```python
from build123d import *
from build123d import SkipClean  # not in build123d's __all__

# Parameters (mm, degrees)
F0_R     = 8.89
F0_R_2   = 5.969
F3_R     = 7.62
F3_R_2   = 5.969
F4_R     = 7.62
F4_R_2   = 5.969
F5_DEPTH = 17.78


with BuildPart() as f2:
    # F2: sweep along a path in F1
    with BuildLine(Plane.XY) as f2_path:
        Line((0, 0), (0, 12.7))
        ThreePointArc((0, 12.7), (12.7, 25.4), (25.4, 12.7))
        Line((25.4, 12.7), (25.4, 0))
    # F0 (on Front) → F2 (sweep)
    with BuildSketch(Plane.XZ):
        Circle(F0_R)
        Circle(F0_R_2, mode=Mode.SUBTRACT)
    sweep(path=f2_path.line)

    # F3 (on face) + F4 (on face) → F5 (join)
    with BuildSketch(Plane.XZ):
        Circle(F3_R)
        Circle(F3_R_2, mode=Mode.SUBTRACT)
    with BuildSketch(Plane.XZ):
        with Locations((25.4, 0)):
            Circle(F4_R)
        with Locations((25.4, 0)):
            Circle(F4_R_2, mode=Mode.SUBTRACT)
    with SkipClean():  # cleaning this boolean's faces spoils the solid; the shape is the same uncleaned
        extrude(amount=F5_DEPTH)


solid = f2.part
```
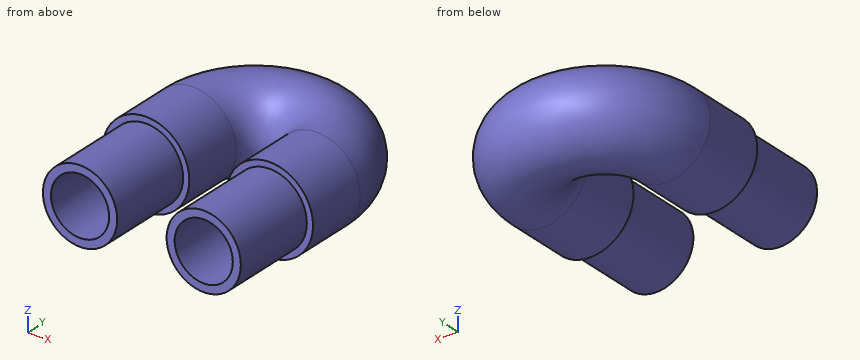
Part model, mm, in its own coordinate system. Give positions to 0.01 mm unless a question says otherwise; leave off trailing zeros. Loops run counter-clockwise (first coordinate to the right, second up) from the corner with the lowest first, then second, coordinate; pieces in that order, holes last. Notation, with made-up numbers: M -21,32.5 L 6,32.5 A16 ccw 6,52.5 Z; hole C -14,51.5 d10. An arc over 180 degrees is marked long. Return JSON: item names as keys, results as strings.
1) Flat gauge pins, fed straight in: pin 1 Ø10 at (x, z) = (5.5, -2.5) entering from +Y; pin 2 Ø1.5 at (x, z) = (28.5, -0.5) entering from -Y; pin 3 Ø6 at (y, z) = (18, -6) entering from +X; pin 4 Ø2 at (x, y) = (9, -3) entering from -Z. Where does each tip first touch, or does it go through?
Calculated:
{"pin 1": "stops at y = 34.12", "pin 2": "stops at y = 21.29", "pin 3": "stops at x = 33.27", "pin 4": "passes through"}
2) Saw through at A-A, the plane z = 0. List the corners of the cut face in (x, y).
Calculated:
{"outline": "M -8.89,0 L -7.62,0 L -7.62,-17.78 L -5.97,-17.78 L -5.97,12.7 A18.67 cw 31.37,12.7 L 31.37,-17.78 L 33.02,-17.78 L 33.02,0 L 34.29,0 L 34.29,12.7 A21.59 ccw -8.89,12.7 Z; M 5.97,-17.78 L 7.62,-17.78 L 7.62,0 L 8.89,0 L 8.89,12.7 A3.81 cw 16.51,12.7 L 16.51,0 L 17.78,0 L 17.78,-17.78 L 19.43,-17.78 L 19.43,12.7 A6.73 ccw 5.97,12.7 Z"}
3) Saw through at C-C, the plane z = 3.5. List the corners of the cut face in (x, y).
Calculated:
{"outline": "M -8.17,0 L -6.77,0 L -6.77,-17.78 L -4.84,-17.78 L -4.84,12.7 A17.54 cw 30.24,12.7 L 30.24,-17.78 L 32.17,-17.78 L 32.17,0 L 33.57,0 L 33.57,12.7 A20.87 ccw -8.17,12.7 Z; M 4.84,-17.78 L 6.77,-17.78 L 6.77,0 L 8.17,0 L 8.17,12.7 A4.53 cw 17.23,12.7 L 17.23,0 L 18.63,0 L 18.63,-17.78 L 20.56,-17.78 L 20.56,12.7 A7.86 ccw 4.84,12.7 Z"}
4) Drill centre lines: line 1 (X direction, y = 3, z = 1.25); line 2 (X direction, y = -2, z = 3.25); line 3 (X direction, y = 18.5, z = -1). Where is each one in solid material? Low to high.
Calculated:
{"line 1": "x = -8.8 to -5.84, 5.84 to 8.8, 16.6 to 19.56, 31.24 to 34.2", "line 2": "x = -6.89 to -5.01, 5.01 to 6.89, 18.51 to 20.39, 30.41 to 32.29", "line 3": "x = -8.04 to -4.96, 9.12 to 16.28, 30.36 to 33.44"}
5) Saw through at B-B, the plane y = 11. List the corners of the cut face in (x, z).
Calculated:
{"outline": "C 0,0 d17.78; C 25.4,0 d17.78; hole C 0,0 d11.94; hole C 25.4,0 d11.94"}
